Source: CAD feature listing. Evaluate the final solid. Frame: model axes, mm. Face numbers are marked on the shaded views. A direction names the side the tool comes from. Round coordinates to 2 decimals unless told otherwise and drop trailing zeros. Order: outer loops, then holes, each group sorted by start corner. A loop starts at its lowest first (then second) coordinate and runs counter-clockwise, first axis right, second up. Notation, with made-up numbers: (-7.75, -18.5) - (39.25, -18.5) arc R27 cw to (39.25, 14.5) - close; hole circle Ø6 at (-11, 23.25). An arc over 180 degrees is marked (long way). Use one line per item in the form item = value. Start each with the question number.
Q1. Cut plane C-C, the plane y = -4.5. Return the cut outline in (x, z), and give its area (3 significant figures).
Q2. Ray query, line 1 (Y direction, x = -1.5, z = 4); line 2 (Z direction, x = -0.5, y = -2.75). Return the intervals inside material, ascending. Write a range as [from, to].
Q3. Cut plane B-B, the plane x = 3.5. Return the cut outline in (y, z), and give its area (3 significant figures).
Q4. Cut plane D-D, the plane y = 2. Return the cut outline in (x, z).
Q5. Cut plane A-A, the plane z = 3.5. Return the cut outline in (x, y), and give its area (3 significant figures).
Q6. Set-up query: the marked faces 1 and 2. Return all of +Z, -Z, +X, -X, +Y, -Y with unobstructed straight access to the full face (end or side cutting, diameter ignored); none if empty.
Q7. Draft query along Y for the marked faces 3, 4 and 5. Return one class per face: released by +Y, released by -Y, zero draft, split by the parting line, or undercut.
Q8. Pin query (flat end, axial travel): pin 1 Ø1 at (x, z) = (1, 6) entering from -Y; pin 2 Ø2.5 at (y, z) = (0, 3) entering from +X; pin 3 Ø1 at (x, y) = (3.5, -4) entering from -Z. Return the tip coordinate at first contact, or that it passes through.
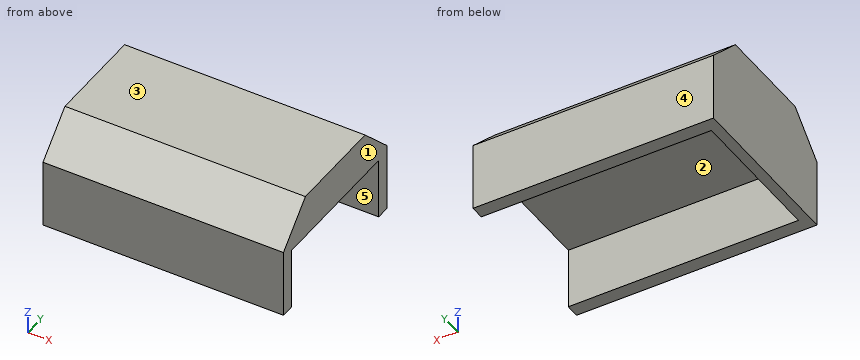
from build123d import *

# Parameters (mm, degrees)
F0_W     = 17.78
F0_H     = 12.7
F1_DEPTH = 5.08
F3_DEPTH = 17.78
F4_W     = 10.668
F4_H     = 4.572
F5_DEPTH = 17.018


with BuildPart() as f1:
    # F0 (on Top) → F1 (new body)
    with BuildSketch(Plane.XY):
        Rectangle(F0_W, F0_H)
    extrude(amount=F1_DEPTH)

    # F2 (on face) → F3 (join)
    with BuildSketch(Plane.YZ.offset(8.89)):
        Polygon((-3.655923, 7.774077), (-6.35, 5.08), (6.35, 5.08), (3.655923, 7.774077), (0, 7.774077), align=None)
    extrude(amount=-F3_DEPTH)

    # F4 (on face) → F5 (cut)
    with BuildSketch(Plane.YZ.offset(8.89)):
        with Locations((0, 2.286)):
            Rectangle(F4_W, F4_H)
    extrude(amount=-F5_DEPTH, mode=Mode.SUBTRACT)


solid = f1.part
Completed:
q1.outline = (-8.89, 0) - (-8.13, 0) - (-8.13, 4.57) - (8.89, 4.57) - (8.89, 6.93) - (-8.89, 6.93) - close
q1.area = 45.4 mm2
q2.line_1 = [-6.35, -5.33], [5.33, 6.35]
q2.line_2 = [4.57, 7.77]
q3.outline = (-6.35, 0) - (-5.33, 0) - (-5.33, 4.57) - (5.33, 4.57) - (5.33, 0) - (6.35, 0) - (6.35, 5.08) - (3.66, 7.77) - (-3.66, 7.77) - (-6.35, 5.08) - close
q3.area = 42.7 mm2
q4.outline = (-8.89, 0) - (-8.13, 0) - (-8.13, 4.57) - (8.89, 4.57) - (8.89, 7.77) - (-8.89, 7.77) - close
q5.outline = (-8.89, -6.35) - (8.89, -6.35) - (8.89, -5.33) - (-8.13, -5.33) - (-8.13, 5.33) - (8.89, 5.33) - (8.89, 6.35) - (-8.89, 6.35) - close
q5.area = 44.3 mm2
q6.face_1 = +Z, -Z, +X, +Y, -Y
q6.face_2 = -Z, +X
q7.face_3 = zero draft
q7.face_4 = released by +Y
q7.face_5 = undercut
q8.pin_1 = -5.93
q8.pin_2 = -8.13
q8.pin_3 = 4.57
